Autodesk Inventor part; units mm, degrees
ref_plane "YZ Plane" through (0, 0, 0) normal (1, 0, 0) x (0, 1, 0)
ref_plane "XZ Plane" through (0, 0, 0) normal (0, 1, 0) x (-1, 0, 0)
ref_plane "XY Plane" through (0, 0, 0) normal (0, 0, 1) x (1, 0, 0)
sketch "Sketch1" plane through (0, 0, 0) normal (0, 0, 1) x (1, 0, 0)
  line L0 (0, 0) -> (25.4, 0)
  line L1 (25.4, 0) -> (25.4, 50.8)
  line L2 (25.4, 50.8) -> (0, 50.8)
  line L3 (0, 50.8) -> (0, 0)
  line L4 (1.5875, 49.2125) -> (23.8125, 49.2125)
  line L5 (23.8125, 49.2125) -> (23.8125, 1.5875)
  line L6 (23.8125, 1.5875) -> (1.5875, 1.5875)
  line L7 (1.5875, 1.5875) -> (1.5875, 49.2125)
  dimension "d0" = 25.4
  dimension "d1" = 50.8
  dimension "d2" = 1.5875
extrude "Extrusion1" add sketch "Sketch1" along normal blind 685.8
sketch "Sketch2" plane through (0, 50.8, 0) normal (0, 1, 0) x (1, 0, 0)
  line L0 (23.8125, 0) -> (1.5875, 0) construction
  line L1 (12.7, 0) -> (12.7, -12.7) construction
  line L2 (12.7, -12.7) -> (12.7, -38.1) construction
  line L3 (12.7, -38.1) -> (12.7, -63.5) construction
  line L4 (12.7, -63.5) -> (12.7, -88.9) construction
  line L5 (12.7, -88.9) -> (12.7, -114.3) construction
  line L6 (12.7, -114.3) -> (12.7, -139.7) construction
  line L7 (12.7, -139.7) -> (12.7, -165.1) construction
  line L8 (12.7, -165.1) -> (12.7, -190.5) construction
  line L9 (12.7, -190.5) -> (12.7, -215.9) construction
  line L10 (12.7, -215.9) -> (12.7, -241.3) construction
  line L11 (12.7, -241.3) -> (12.7, -266.7) construction
  line L12 (12.7, -266.7) -> (12.7, -292.1) construction
  line L13 (12.7, -292.1) -> (12.7, -317.5) construction
  line L14 (12.7, -317.5) -> (12.7, -342.9) construction
  line L15 (12.7, -342.9) -> (12.7, -368.3) construction
  line L16 (12.7, -368.3) -> (12.7, -393.7) construction
  line L17 (12.7, -393.7) -> (12.7, -419.1) construction
  line L18 (12.7, -419.1) -> (12.7, -444.5) construction
  line L19 (12.7, -444.5) -> (12.7, -469.9) construction
  line L20 (12.7, -469.9) -> (12.7, -495.3) construction
  line L21 (12.7, -495.3) -> (12.7, -469.9) construction
  line L22 (12.7, -469.9) -> (12.7, -495.3) construction
  line L23 (12.7, -495.3) -> (12.7, -520.7) construction
  line L24 (12.7, -520.7) -> (12.7, -546.1) construction
  line L25 (12.7, -546.1) -> (12.7, -571.5) construction
  line L26 (12.7, -571.5) -> (12.7, -596.9) construction
  line L27 (12.7, -596.9) -> (12.7, -622.3) construction
  line L28 (12.7, -622.3) -> (12.7, -647.7) construction
  line L29 (12.7, -647.7) -> (12.7, -673.1) construction
  circle A0 centre (12.7, -673.1) radius 2.5781
  circle A1 centre (12.7, -647.7) radius 2.5781
  circle A2 centre (12.7, -622.3) radius 2.5781
  circle A3 centre (12.7, -596.9) radius 2.5781
  circle A4 centre (12.7, -571.5) radius 2.5781
  circle A5 centre (12.7, -546.1) radius 2.5781
  circle A6 centre (12.7, -520.7) radius 2.5781
  circle A7 centre (12.7, -495.3) radius 2.5781
  circle A8 centre (12.7, -469.9) radius 2.5781
  circle A9 centre (12.7, -444.5) radius 2.5781
  circle A10 centre (12.7, -419.1) radius 2.5781
  circle A11 centre (12.7, -393.7) radius 2.5781
  circle A12 centre (12.7, -368.3) radius 2.5781
  circle A13 centre (12.7, -342.9) radius 2.5781
  circle A14 centre (12.7, -317.5) radius 2.5781
  circle A15 centre (12.7, -292.1) radius 2.5781
  circle A16 centre (12.7, -266.7) radius 2.5781
  circle A17 centre (12.7, -241.3) radius 2.5781
  circle A18 centre (12.7, -215.9) radius 2.5781
  circle A19 centre (12.7, -190.5) radius 2.5781
  circle A20 centre (12.7, -165.1) radius 2.5781
  circle A21 centre (12.7, -139.7) radius 2.5781
  circle A22 centre (12.7, -114.3) radius 2.5781
  circle A23 centre (12.7, -88.9) radius 2.5781
  circle A24 centre (12.7, -63.5) radius 2.5781
  circle A25 centre (12.7, -38.1) radius 2.5781
  circle A26 centre (12.7, -12.7) radius 2.5781
  point P0 (0, 0)
  dimension "d5" = 12.7
  dimension "d6" = 25.4
  dimension "d7" = 25.4
  dimension "d8" = 25.4
  dimension "d9" = 25.4
  dimension "d10" = 25.4
  dimension "d11" = 25.4
  dimension "d12" = 25.4
  dimension "d13" = 25.4
  dimension "d14" = 25.4
  dimension "d15" = 25.4
  dimension "d16" = 25.4
  dimension "d17" = 25.4
  dimension "d18" = 25.4
  dimension "d19" = 25.4
  dimension "d20" = 25.4
  dimension "d21" = 25.4
  dimension "d22" = 25.4
  dimension "d23" = 25.4
  dimension "d24" = 25.4
  dimension "d25" = 25.4
  dimension "d26" = 25.4
  dimension "d27" = 25.4
  dimension "d28" = 25.4
  dimension "d29" = 25.4
  dimension "d30" = 25.4
  dimension "d31" = 25.4
  dimension "d32" = 25.4
  dimension "d33" = 25.4
  dimension "d34" = 5.1562
  dimension "d35" = 5.1562
  dimension "d36" = 5.1562
  dimension "d37" = 5.1562
  dimension "d38" = 5.1562
  dimension "d39" = 5.1562
  dimension "d40" = 5.1562
  dimension "d41" = 5.1562
  dimension "d42" = 5.1562
  dimension "d43" = 5.1562
  dimension "d44" = 5.1562
  dimension "d45" = 5.1562
  dimension "d46" = 5.1562
  dimension "d47" = 5.1562
  dimension "d48" = 5.1562
  dimension "d49" = 5.1562
  dimension "d50" = 5.1562
  dimension "d51" = 5.1562
  dimension "d52" = 5.1562
  dimension "d53" = 5.1562
  dimension "d54" = 5.1562
  dimension "d55" = 5.1562
  dimension "d56" = 5.1562
  dimension "d57" = 5.1562
  dimension "d58" = 5.1562
  dimension "d59" = 5.1562
  dimension "d60" = 5.1562
extrude "Extrusion2" cut sketch "Sketch2" against normal blind 685.8
sketch "Sketch3" plane through (0, 50.8, 0) normal (0, 1, 0) x (1, 0, 0)
  line L0 (0, 0) -> (25.4, 0)
  line L1 (0, 0) -> (69.85, 0)
  line L2 (69.85, 0) -> (69.85, -50.8)
  line L3 (69.85, -50.8) -> (0, -50.8)
  line L4 (0, -50.8) -> (0, 0)
  line L5 (0, -685.8) -> (25.4, -685.8)
  line L6 (0, -685.8) -> (104.9991, -685.8)
  line L7 (104.9991, -685.8) -> (104.9991, -660.4)
  line L8 (104.9991, -660.4) -> (0, -660.4)
  line L9 (0, -660.4) -> (0, -685.8)
  dimension "d63" = 69.85
  dimension "d64" = 50.8
  dimension "d65" = 25.4
extrude "Extrusion3" cut sketch "Sketch3" against normal blind 50.8
properties part number "Front and Back Bar"
CAD build for the part. Positions are in the model's coordinates, mm. A direction names the side the tool comes from. Coordinates: 2 decimals unless noted, no trailing zeros. Write each loop counter-clockwise with the first axis right and the second up, starting at its lowest first coordinate (ties: lowest second). Pieces come first, ordered by that corner, then holes. Notation, with made-up numbers: (12.25, -16.5) -> (64.25, -16.5) arc R25 cw to (64.25, -2.5) -> close; hole circle Ø4 at (1.25, 39.5). An arc over 180 degrees is marked (long way). Return JSON: item names as keys, results as strings. Group by question number.
Q1. Pull direction Y, two halves, no side cores. Call faces 3 (the face through (13, 0, 351)), 4 (the face through (1.588, 25, 351)), 5 (the face through (24, 27, 660.4)): released by +Y, released by -Y, zero draft, split by the parting line, or undercut.
Q2. Cut at A-A, the plane y = 32. Give the cut face in (x, z).
Q3. Which spindle directions (+Z, -Z, +X, -X, +Y, -Y) get a long thin tool onto all of the face, cutting with end or side? Do faces 1 (the face through (13, 1.588, 351)), 2 (the face through (0, 26, 351)). Say none if no direction does.
Q4. Flat gauge pin, fed straight in: pin 1 (4 mm diameter, centred on y = 40.5, z = 169, fed in from -X). Where does the tip first touch, or does it go through?
Q5. Drill centre lines: line 1 (Y direction, x = 22.75, z = 343); line 2 (X direction, y = 50.1, z = 469.9); line 3 (X direction, y = 38, z = 448.5). Where is each one in solid material? Low to high.
Q6. Cut at B-B, the plane z = 430. Give the cut face in (x, y), then the cut area to 3 significant figures.
Returned:
{
 "1": {"face 3": "released by -Y", "face 4": "undercut", "face 5": "zero draft"},
 "2": {"outline": "(0, 50.8) -> (1.59, 50.8) -> (1.59, 660.4) -> (0, 660.4) -> close; (23.81, 50.8) -> (25.4, 50.8) -> (25.4, 660.4) -> (23.81, 660.4) -> close"},
 "3": {"face 1": "+Z, -Z", "face 2": "+Z, -Z, -X, +Y, -Y"},
 "4": {"pin 1": "stops at x = 0"},
 "5": {"line 1": "y = 0 to 1.59, 49.21 to 50.8", "line 2": "x = 0 to 10.12, 15.28 to 25.4", "line 3": "x = 0 to 1.59, 23.81 to 25.4"},
 "6": {"outline": "(0, 0) -> (25.4, 0) -> (25.4, 50.8) -> (0, 50.8) -> close; hole (1.59, 1.59) -> (23.81, 1.59) -> (23.81, 49.21) -> (1.59, 49.21) -> close", "area": "232 mm2"}
}
